```python
from build123d import *

# Parameters (mm, degrees)
SKETCH1_R               = 7.9375
OUTER_CIRCLE_DEPTH      = 6.35
TOOTH_CUT_DEPTH         = 13.896910967
TEETH_PATTERN_COUNT     = 18
CUT_EXTRUDE1_DEPTH      = 12.621761341
CUT_EXTRUDE1_DEPTH_BACK = 12.621761341
PITCH_DIAMETER_R        = 4.826


with BuildPart() as part:
    # Sketch1 → Outer Circle (new body)
    with BuildSketch(Plane.XY):
        Circle(SKETCH1_R)
    extrude(amount=OUTER_CIRCLE_DEPTH)

    # Sketch2 → Tooth Cut (cut, through all)
    with BuildSketch(Plane.XY.offset(6.35)):
        with BuildLine():
            ThreePointArc((-0.452232993, 6.333876011), (0, 6.35), (0.452232993, 6.333876011))
            ThreePointArc((0.452232993, 6.333876011), (0.624488533, 7.142351531), (1.011484471, 7.872788922))
            ThreePointArc((1.011484471, 7.872788922), (0, 7.9375), (-1.011484471, 7.872788922))
            ThreePointArc((-1.011484471, 7.872788922), (-0.624488533, 7.142351531), (-0.452232993, 6.333876011))
        make_face()
    tooth_cut = extrude(amount=-TOOTH_CUT_DEPTH, mode=Mode.SUBTRACT)

    # Teeth Pattern: Tooth Cut ×18 about axis
    teeth_pattern_axis = Axis((0, 0, 0), (0, 0, 1))
    for i in range(1, TEETH_PATTERN_COUNT):
        add(tooth_cut.rotate(teeth_pattern_axis, i * 360 / TEETH_PATTERN_COUNT), mode=Mode.SUBTRACT)

    # Pitch Diameter → Cut-Extrude1 (cut, two sides: drawn at the far end of the back side and taken through both)
    with BuildSketch(Plane.XY.offset(3.175).offset(-CUT_EXTRUDE1_DEPTH_BACK)):
        Circle(PITCH_DIAMETER_R)
    extrude(amount=CUT_EXTRUDE1_DEPTH + CUT_EXTRUDE1_DEPTH_BACK, mode=Mode.SUBTRACT)


solid = part.part
```
Model file for the job. Use its own axes, mm. A direction names the side the tool comes from. Coordinates: 2 decimals unless noted, no trailing zeros. Loops run counter-clockwise (first coordinate to the right, second up) from the corner with the lowest first, then second, coordinate; pieces in that order, holes last. Notation, with made-up numbers: (-24.75, 59) -> (8.25, 59) arc R19 ccw to (8.25, 65) -> close; hole circle Ø9 at (62.5, -30). An arc over 180 degrees is marked (long way). Answer as a JSON object with one key per item and string values.
Q1. 3-axis set-ups, long thin cutter, end or side, ignore diameter. For faces 1 (the cylindrical face through (0.62, 7.13, 3.22)), 2 (the cylindrical face through (-6.935, -1.861, 3.219)), 3 (the cylindrical face through (-5.059, -5.064, 3.219)), 4 (the cylindrical face through (7.154, -0.623, 3.219)): which of +Z, -Z, +X, -X, +Y, -Y reach the whole face in a straight line?
Report:
{"face 1": "+Z, -Z, +Y", "face 2": "+Z, -Z, -X", "face 3": "+Z, -Z, -Y", "face 4": "+Z, -Z"}
Q2. Flat gauge pins, fed straight in: P1, Ø1.5, axis at y = -5, z = 5, coming from the -X side; P2, Ø3, axis at x = 6, z = 5, coming from the -Y side. Where does each tip first touch, or does it go through?
Report:
{"P1": "stops at x = -6.31", "P2": "stops at y = -5.38"}
Q3. Probe probe 1 along X at (y, z) = (0, 3); probe 2 along Y at (x, z) = (0, 1.5); probe 3 along X at (y, z) = (6.5, 0.5). List the from-to ranges inside material, lowest first.
Report:
{"probe 1": "x = -7.94 to -4.83, 4.83 to 7.94", "probe 2": "y = -6.35 to -4.83, 4.83 to 6.35", "probe 3": "x = -4.27 to -3.03, -1.83 to -0.47, 0.47 to 1.83, 3.03 to 4.27"}
Q4. Cut at B-B (x = 0). List the corners of the cut face in (y, z).
Report:
{"outline": "(-6.35, 0) -> (-4.83, 0) -> (-4.83, 6.35) -> (-6.35, 6.35) -> close; (4.83, 0) -> (6.35, 0) -> (6.35, 6.35) -> (4.83, 6.35) -> close"}
Q5. Cut at A-A (y = 0). List the corners of the cut face in (x, z), and give its area (3 significant figures).
Report:
{"outline": "(-7.94, 0) -> (-4.83, 0) -> (-4.83, 6.35) -> (-7.94, 6.35) -> close; (4.83, 0) -> (7.94, 0) -> (7.94, 6.35) -> (4.83, 6.35) -> close", "area": "39.5 mm2"}
Q6. Pull direction X, two halves, no side cores. Call faces 5 (the cylindrical face through (-0.01, 6.35, 3.22)), 6 (the flat face through (-1, 5, 6.35)), 7 (the cylindrical face through (6.92, -1.85, 3.22)): released by +X, released by -X, zero draft, split by the parting line, or undercut.
Report:
{"face 5": "undercut", "face 6": "zero draft", "face 7": "released by +X"}
Q7. Cut at C-C (x = -4). List the corners of the cut face in (y, z) (3 decimals), and give its area (3 significant figures).
Report:
{"outline": "(-6.856, 0) -> (-5.605, 0) -> (-5.605, 6.35) -> (-6.856, 6.35) -> close; (-4.932, 0) -> (-2.7, 0) -> (-2.7, 6.35) -> (-4.932, 6.35) -> close; (2.7, 0) -> (4.932, 0) -> (4.932, 6.35) -> (2.7, 6.35) -> close; (5.605, 0) -> (6.856, 0) -> (6.856, 6.35) -> (5.605, 6.35) -> close", "area": "44.2 mm2"}
